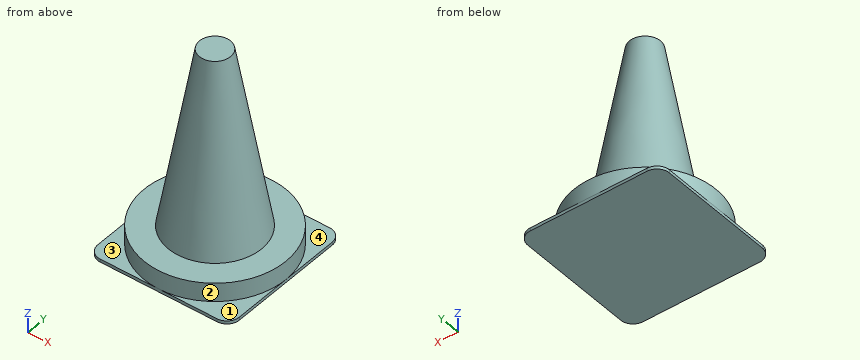
from build123d import *

# Parameters (mm, degrees)
PAD_DEPTH    = 5
SKETCH001_R  = 114
PAD001_DEPTH = 30
SKETCH002_R  = 75
SKETCH003_R  = 25


with BuildPart() as part:
    # Sketch → Pad (new body)
    with BuildSketch(Plane.XY):
        with BuildLine():
            Line((-94, -114), (94, -114))
            ThreePointArc((94, -114), (108.142136, -108.142136), (114, -94))
            Line((114, -94), (114, 94))
            ThreePointArc((114, 94), (108.142136, 108.142136), (94, 114))
            Line((94, 114), (-94, 114))
            ThreePointArc((-94, 114), (-108.142136, 108.142136), (-114, 94))
            Line((-114, 94), (-114, -94))
            ThreePointArc((-114, -94), (-108.142136, -108.142136), (-94, -114))
        make_face()
    extrude(amount=PAD_DEPTH)

    # Sketch001 (on Face10 of Pad) → Pad001 (join)
    with BuildSketch(Plane.XY.offset(5)):
        Circle(SKETCH001_R)
    extrude(amount=PAD001_DEPTH)

    # Sketch002 (on Face15 of Pad001) → AdditiveLoft section 0
    with BuildSketch(Plane.XY.offset(35)):
        Circle(SKETCH002_R)
    # Sketch003 (on DatumPlane) → AdditiveLoft section 1
    with BuildSketch(Plane.XY.offset(325)):
        Circle(SKETCH003_R)
    loft()


solid = part.part
Geometry check sheet. Reference: the model listing, model coordinates, mm. Face numbers are marked on the shaded views. A direction names the side the tool comes from. Give positions to 0.01 mm unless a question says otherwise; leave off trailing zeros. Write each loop counter-clockwise with the first axis right and the second up, starting at its lowest first coordinate (ties: lowest second). Pieces come first, ordered by that corner, then holes.
1) Cross-section at A-A (z = 102.5). Record the boundary of the cut face in (x, y), plus the area to 3 significant figures.
Values follow:
outline: circle Ø126.72 at (0, 0)
area: 12,600 mm2
2) Go/stop test with flat-tipped pins: pin 1 Ø2 at (x, y) = (-30.5, -87.5) entering from +Z; pin 2 Ø6 at (x, z) = (-15, 96) entering from +Y; pin 3 Ø12 at (x, z) = (15, 92) entering from -Y. Record where each tip stops, or that it passes through.
Values follow:
pin 1: stops at z = 35
pin 2: stops at y = 63.56
pin 3: stops at y = -65.02
3) Thickness scan on line 1 (Z direction, x = -31, y = 84); line 2 (X direction, y = 1.5, z = 190); line 3 (Y direction, x = 2.5, z = 192). Record the ranges inside material, lowest first.
Values follow:
line 1: z = 0 to 35
line 2: x = -48.25 to 48.25
line 3: y = -47.87 to 47.87
4) Set-up check for the marked faces 1, 2, 3 and 4: record each of +Z, -Z, +X, -X, +Y, -Y from which the full face is reachable in a straight line by a thin tool's end or side.
Values follow:
face 1: +Z, +X, -Y
face 2: +Z
face 3: +Z, -X, -Y
face 4: +Z, +X, +Y
